Build history of the part. All positions in model axes, mm. Face numbers are marked on the shaded views. A direction names the side the tool comes from. Give positions to 0.01 mm unless a question says otherwise; leave off trailing zeros. Loops run counter-clockwise (first coordinate to the right, second up) from the corner with the lowest first, then second, coordinate; pieces in that order, holes last.
1) Two-plate mould, pull along X, no slides. Class the marked faces 5, 6, 7 and 8: +X half, -X half, draft (parallel to the pull), parting line (faces both ways), or undercut.
2) Band-saw the part on B-B on z = 0. List the corners of the cut face in (x, y).
3) Wall check: line 1 (Z direction, x = -13, y = -1.4); line 2 (Z direction, x = 3.5, y = -0.9); line 3 (X direction, y = -3.7, z = -11). Give the ranges that are in metal, low to high.
4) Band-saw the part on A-A on x = 0.25. List the corners of the cut face in (y, z), then the cut area to 3 significant figures.
5) 3-axis set-ups, long thin cutter, end or side, ignore diameter. For the marked faces 1, 2, 3 and 4: which of +Z, -Z, +X, -X, +Y, -Y reach the whole face in a straight line?
6) Flat gauge pins, fed straight in: P1, Ø1.5, axis at x = 1.5, y = -1.5, coming from the -Z side; P2, Ø1.5, axis at y = -3.5, z = -1, coming from the -X side. Where does each tip first touch, or does it go through?
```python
from build123d import *

# Parameters (mm, degrees)
F1_DEPTH = 4
F2_COUNT = 24


with BuildPart() as f1:
    # F0 (on Front) → F1 (new body)
    with BuildSketch(Plane.XZ):
        Polygon((5.1303021499, 14.0953893118), (0, 13), (1.7364817767, 9.8480775301), (1.3911704768, 7.889719833), (5, 8.6602540378), (4.4462618632, 12.2160040702), align=None)
    extrude(amount=F1_DEPTH)

    # F2: F1 ×24 about axis
    f2_axis = Axis((0, 0, 0), (0, -1, 0))


with BuildPart() as f1_1:
    add(f1.part)
    for i in range(1, F2_COUNT):
        add(f1.part.rotate(f2_axis, i * 360 / F2_COUNT))


solid = f1_1.part
```
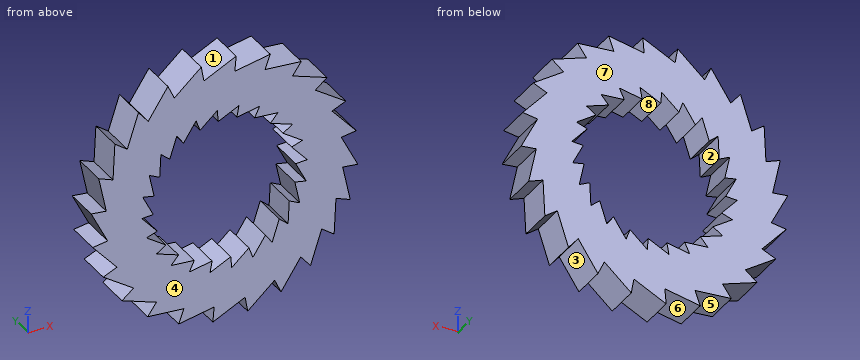
Findings below:
1. face 5: -X half
1. face 6: undercut
1. face 7: draft
1. face 8: undercut
2. outline: (-14.28, -4) - (-8.34, -4) - (-8.34, 0) - (-14.28, 0) - close; (8.34, -4) - (14.28, -4) - (14.28, 0) - (8.34, 0) - close
3. line 1: z = -6.72 to -6.06, -4.57 to 4.73
3. line 2: z = -13.96 to -8.25, 7.25 to 7.51, 8.34 to 13.75
3. line 3: x = -7.7 to 8.02, 9.23 to 9.8
4. outline: (-4, -14.15) - (0, -14.15) - (0, -8.21) - (-4, -8.21) - close; (-4, 8.47) - (0, 8.47) - (0, 14.4) - (-4, 14.4) - close
4. area: 47.5 mm2
5. face 1: +Z, +Y, -Y
5. face 2: +Y, -Y
5. face 3: -Z, +Y, -Y
5. face 4: +Z, -Z, +X, -X, -Y
6. P1: stops at z = -13.89
6. P2: stops at x = -14.15
